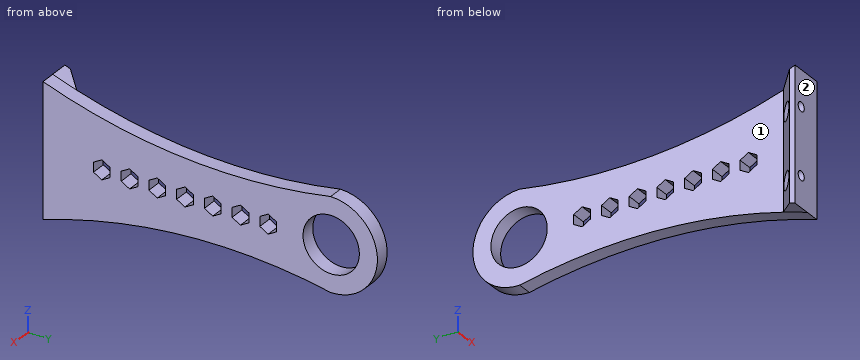
Autodesk Inventor part; units mm, degrees
ref_plane "YZ Plane" through (0, 0, 0) normal (1, 0, 0) x (0, 1, 0)
ref_plane "XZ Plane" through (0, 0, 0) normal (0, 1, 0) x (-1, 0, 0)
ref_plane "XY Plane" through (0, 0, 0) normal (0, 0, 1) x (1, 0, 0)
sketch "Sketch1" plane through (0, 0, 0) normal (1, 0, 0) x (0, 1, 0)
  line L0 (0, 0) -> (155.9349, 0)
  circle A0 centre (155.9349, 0) radius 15.25
  circle A1 centre (155.9349, 0) radius 25
  line L1 (155.6119, 24.9979) -> (0, 35.995)
  line L2 (0, 0) -> (0, 35.995)
  line L3 (155.6119, -24.9979) -> (0, -35.995)
  line L4 (0, 0) -> (0, -35.995)
  arc A2 (0, 35.995) -> (155.6119, 24.9979) centre (98.1634, 318.5597) ccw
  arc A3 (155.6119, -24.9979) -> (0, -35.995) centre (98.1634, -318.5597) ccw
  point P0 (155.6119, -24.9979)
  dimension "d2" = 50
  dimension "d0" = 155.9349
  dimension "d1" = 30.5
  dimension "d3" = 156
extrude "Extrusion1" add sketch "Sketch1" along normal blind 8 contours L2 A2 A1 L0 | L0 A1 A3 L4 | A1 A2 A3
sketch "Sketch2" plane through (0, 0, 0) normal (-1, 0, 0) x (0, 0, 1)
  arc A0 (24.9979, 155.6119) -> (-24.9979, 155.6119) centre (0, 155.9349) ccw
  arc A1 (-35.995, 0) -> (-24.9979, 155.6119) centre (-318.5597, 98.1634) ccw
  line L0 (35.995, 0) -> (-35.995, 0)
  arc A2 (24.9979, 155.6119) -> (35.995, 0) centre (318.5597, 98.1634) ccw
  circle A3 centre (0, 155.9349) radius 15.25
  line L1 (0, 0) -> (0, 13)
  line L2 (0, 13) -> (-31.8089, 13)
  arc A4 (-35.995, 0) -> (-24.9979, 155.6119) centre (-318.5597, 98.1634) ccw
  line L3 (0, 13) -> (31.8089, 13)
  arc A5 (24.9979, 155.6119) -> (35.995, 0) centre (318.5597, 98.1634) ccw
  point P0 (-31.8089, 13)
  point P1 (31.8089, 13)
  dimension "d6" = 13
extrude "Extrusion2" add sketch "Sketch2" along normal blind 10 contours A2 L0 L1 L3 | L2 L1 L0 A1
chamfer "Chamfer1" distance 10 angle 45 1 edges at (-10, 13, 0)
sketch "Sketch3" plane through (0, 0, 0) normal (-1, 0, 0) x (0, 0, 1)
  line L0 (-31.8089, 13) -> (31.8089, 13)
  line L1 (0, 13) -> (0, 140.6849)
  circle A0 centre (0, 155.9349) radius 15.25
  line L2 (-5.2273, 76.8425) -> (-2.6137, 81.3695)
  line L3 (-2.6137, 81.3695) -> (2.6137, 81.3695)
  line L4 (2.6137, 81.3695) -> (5.2273, 76.8425)
  line L5 (5.2273, 76.8425) -> (2.6137, 72.3155)
  line L6 (2.6137, 72.3155) -> (-2.6137, 72.3155)
  line L7 (-2.6137, 72.3155) -> (-5.2273, 76.8425)
  line L8 (-5.2273, 91.8425) -> (-2.6137, 96.3695)
  line L9 (-2.6137, 96.3695) -> (2.6137, 96.3695)
  line L10 (2.6137, 96.3695) -> (5.2273, 91.8425)
  line L11 (5.2273, 91.8425) -> (2.6137, 87.3155)
  line L12 (2.6137, 87.3155) -> (-2.6137, 87.3155)
  line L13 (-2.6137, 87.3155) -> (-5.2273, 91.8425)
  line L14 (-5.2273, 106.8425) -> (-2.6137, 111.3695)
  line L15 (-2.6137, 111.3695) -> (2.6137, 111.3695)
  line L16 (2.6137, 111.3695) -> (5.2273, 106.8425)
  line L17 (5.2273, 106.8425) -> (2.6137, 102.3155)
  line L18 (2.6137, 102.3155) -> (-2.6137, 102.3155)
  line L19 (-2.6137, 102.3155) -> (-5.2273, 106.8425)
  line L20 (-5.2273, 121.8425) -> (-2.6137, 126.3695)
  line L21 (-2.6137, 126.3695) -> (2.6137, 126.3695)
  line L22 (2.6137, 126.3695) -> (5.2273, 121.8425)
  line L23 (5.2273, 121.8425) -> (2.6137, 117.3155)
  line L24 (2.6137, 117.3155) -> (-2.6137, 117.3155)
  line L25 (-2.6137, 117.3155) -> (-5.2273, 121.8425)
  line L26 (-2.6137, 66.3695) -> (2.6137, 66.3695)
  line L27 (-5.2273, 61.8425) -> (-2.6137, 66.3695)
  line L28 (2.6137, 66.3695) -> (5.2273, 61.8425)
  line L29 (-2.6137, 57.3155) -> (-5.2273, 61.8425)
  line L30 (5.2273, 61.8425) -> (2.6137, 57.3155)
  line L31 (2.6137, 57.3155) -> (-2.6137, 57.3155)
  line L32 (-2.6137, 51.3695) -> (2.6137, 51.3695)
  line L33 (-5.2273, 46.8425) -> (-2.6137, 51.3695)
  line L34 (2.6137, 51.3695) -> (5.2273, 46.8425)
  line L35 (-2.6137, 42.3155) -> (-5.2273, 46.8425)
  line L36 (5.2273, 46.8425) -> (2.6137, 42.3155)
  line L37 (2.6137, 42.3155) -> (-2.6137, 42.3155)
  line L38 (-2.6137, 36.3695) -> (2.6137, 36.3695)
  line L39 (-5.2273, 31.8425) -> (-2.6137, 36.3695)
  line L40 (2.6137, 36.3695) -> (5.2273, 31.8425)
  line L41 (-2.6137, 27.3155) -> (-5.2273, 31.8425)
  line L42 (5.2273, 31.8425) -> (2.6137, 27.3155)
  line L43 (2.6137, 27.3155) -> (-2.6137, 27.3155)
  line L44 (0, 76.8425) -> (20.7534, 76.8425)
  point P0 (0, 0)
  point P1 (0, 81.3695)
  point P2 (0, 91.8425)
  point P3 (0, 96.3695)
  point P4 (0, 106.8425)
  point P5 (0, 111.3695)
  point P6 (0, 121.8425)
  point P7 (0, 126.3695)
  point P8 (0, 66.3695)
  point P9 (0, 61.8425)
  point P10 (0, 51.3695)
  point P11 (0, 46.8425)
  point P12 (0, 36.3695)
  point P13 (0, 31.8425)
  dimension "d12" = 9.054
  dimension "d15" = 15
  dimension "d22" = 15
extrude "Extrusion3" cut sketch "Sketch3" against normal blind 12 contours L43 L41 L39 L38 L1 | L1 L38 L40 L42 L43 | L24 L25 L20 L21 L1 | L1 L21 L22 L23 L24 | L18 L19 L14 L15 L1 | L1 L15 L16 L17 L18 | L12 L13 L8 L9 L1 | L1 L9 L10 L11 L12 | L6 L7 L2 L3 L1 | L1 L44 L5 L6 | L31 L29 L27 L26 L1 | L1 L26 L28 L30 L31 | L37 L35 L33 L32 L1 | L1 L32 L34 L36 L37 | L1 L3 L4 L44
sketch "Sketch4" plane through (8, 0, -35.995) normal (0, -1, 0) x (1, 0, 0)
  line L0 (-18, 0) -> (0, 0)
  line L1 (0, 71.9901) -> (0, 0)
  line L2 (-18, 71.9901) -> (0, 71.9901)
  line L3 (-18, 0) -> (-18, 71.9901)
  line L4 (-18, 71.9901) -> (-9, 71.9901)
  line L5 (-18, 71.9901) -> (-8, 71.9901)
  line L6 (-8, 0) -> (-8, 71.9901)
  line L7 (-8, 67.8039) -> (-8, 55.4246)
  line L8 (-13, 71.9901) -> (-13, 0)
  line L9 (-8, 33.3814) -> (0, 33.3814)
  line L10 (0, 33.3814) -> (-18, 33.3814)
  line L11 (-13, 71.9901) -> (-13, 33.3814)
  line L12 (-13, 33.3814) -> (-13, 0)
  circle A0 centre (-13, 16.6907) radius 2.5
  circle A1 centre (-13, 52.6857) radius 2.5
  point P0 (-8, 35.995)
  point P1 (-8, 60.9929)
  dimension "d29" = 5
  dimension "d30" = 5
extrude "Extrusion4" cut sketch "Sketch4" against normal blind 20 contours A0 L8 | L8 A0 | A1 L8 | L8 A1
chamfer "Chamfer2" distance 2 angle 45 2 edges at (-7.5, 5.5005, -19.3043) (-7.5, 5.5005, 16.6907)
properties part number "HolderB" material "Acetal Resin, Black"
Can you work these out from the model? Positions are in its coordinate system, mm. Face numbers are marked on the shaded views. Round coordinates to 2 decimals unless told otherwise and drop trailing zeros. Loops run counter-clockwise (first coordinate to the right, second up) from the corner with the lowest first, then second, coordinate; pieces in that order, holes last. Notation, with made-up numbers: (43, -22.75) -> (48, -22.75) arc R14 ccw to (48, -17.75) -> close; hole circle Ø4 at (34, -28). An arc over 180 degrees is marked (long way). One line per item, written item: value. Start each with the question number.
1. If I drill on probe 1 along Z at (x, y) = (-5, 3.5); probe 2 along Z at (x, y) = (4.25, 156.5); probe 3 along X at (y, z) = (59.5, -17.5), over which ranges is the centre line in solid material (lowest first)?
2. If we section it at C-C, the plane z = 0: Give the number of separate pieces and of enclosed holes in the cut face, then the cut area to 3 significant figures.
3. For pin 1 (8 mm diameter, centred on x = -2.5, y = 79.5, fed in from -Z); pin 2 (2 mm diameter, centred on x = -1.5, y = 71.5, fed in from -Z); pin 3 (8 mm diameter, centred on x = -6, z = -22.5, fed in from +Y); pin 4 (6 mm diameter, centred on x = 2, y = 47.5, fed in from -Z), each with a flat end and sliding along its axis, tell me the tip position at first contact or that it passes through.
4. If we mould it in two halves opening along Y, with no side actions, what happens to the marked faces 1 and 2? For each: pulls with the +Y half, pulls with the -Y half, needs draft (parallel to the pull), parting line crosses it, or undercut.
5. If we section it at A-A, the plane y = 34: Write out the boundary of the cut face in (x, z).
Calculated:
1. probe 1: z = -34.8 to -21.8, -16.8 to 14.19, 19.19 to 34.8
1. probe 2: z = -24.99 to -15.24, 15.24 to 24.99
1. probe 3: x = 0 to 8
2. separate pieces: 9
2. enclosed holes: 0
2. area: 776 mm²
3. pin 1: stops at z = -20.22
3. pin 2: passes through
3. pin 3: stops at y = 11
3. pin 4: stops at z = -24.28
4. face 1: needs draft
4. face 2: pulls with the -Y half
5. outline: (0, -26.39) -> (8, -26.39) -> (8, -3.98) -> (0, -3.98) -> close; (0, 3.98) -> (8, 3.98) -> (8, 26.39) -> (0, 26.39) -> close
